Autodesk Inventor part; units mm, degrees
ref_plane "YZ Plane" through (0, 0, 0) normal (1, 0, 0) x (0, 1, 0)
ref_plane "XZ Plane" through (0, 0, 0) normal (0, 1, 0) x (-1, 0, 0)
ref_plane "XY Plane" through (0, 0, 0) normal (0, 0, 1) x (1, 0, 0)
sketch "Sketch1" plane through (0, 0, 0) normal (0, 1, 0) x (-1, 0, 0)
  line L0 (-3.5, -2.0207) -> (-3.5, 2.0207)
  line L1 (-3.5, 2.0207) -> (0, 4.0415)
  line L2 (0, 4.0415) -> (3.5, 2.0207)
  line L3 (3.5, 2.0207) -> (3.5, -2.0207)
  line L4 (3.5, -2.0207) -> (0, -4.0415)
  line L5 (0, -4.0415) -> (-3.5, -2.0207)
  point P0 (0, 0)
  point P1 (0, 0)
  dimension "d0" = 7
extrude "Extrusion1" add sketch "Sketch1" against normal blind 32
chamfer "Chamfer1" distance 0.1 angle 45 12 edges at (-1.75, -32, 3.0311) (1.75, -32, 3.0311) (3.5, -32, 0) (1.75, -32, -3.0311) (-1.75, -32, -3.0311) (-3.5, -32, 0) (1.75, 0, 3.0311) (-1.75, 0, 3.0311) (-3.5, 0, 0) (-1.75, 0, -3.0311) (1.75, 0, -3.0311) (3.5, 0, 0)
sketch "Sketch2" plane through (0, -32, 0) normal (0, -1, 0) x (1, 0, 0)
  circle A0 centre (0, 0) radius 2
  dimension "d6" = 4
extrude "Extrusion2" cut sketch "Sketch2" against normal blind 8
sketch "Sketch3" plane through (0, 0, 0) normal (0, 1, 0) x (1, 0, 0)
  circle A0 centre (0, 0) radius 2
  dimension "d9" = 4
extrude "Extrusion3" cut sketch "Sketch3" against normal blind 8
chamfer "Chamfer2" distance 0.2 angle 45 2 edges at (-2, 0, 0) (-2, -32, 0)
thread "Thread1"
thread "Thread2"
properties part number "09-0001" material "Aluminum 6061"
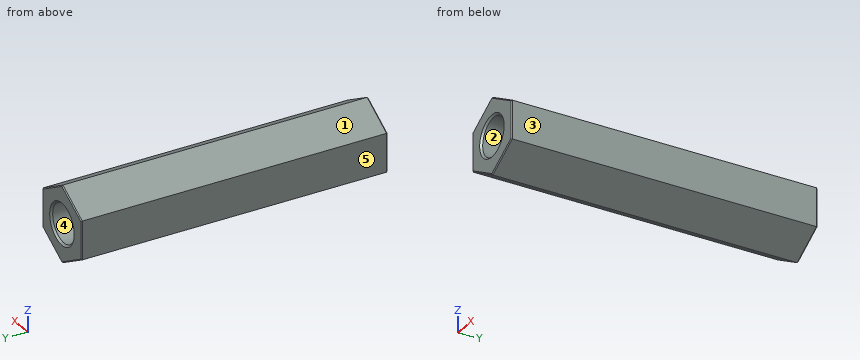
CAD build for the part. Positions are in the model's coordinates, mm. Face numbers are marked on the shaded views. A direction names the side the tool comes from. Round coordinates to 2 decimals unless told otherwise and drop trailing zeros. Order: outer loops, then holes, each group sorted by start corner. A loop starts at its lowest first (then second) coordinate and runs counter-clockwise, first axis right, second up. Notation, with made-up numbers: (13, 22) - (53, 22) arc R32 ccw to (53, 52) - close; hole circle Ø8 at (22.25, 7.5). An arc over 180 degrees is marked (long way). Return JSON: item names as keys, results as strings.
(1) Pin check, flat tips, straight feed: pin 1 Ø2 at (x, z) = (-0.5, -0.5) entering from +Y; pin 2 Ø3.5 at (x, z) = (0, 0) entering from -Y; pin 3 Ø1.5 at (x, y) = (-1.5, -16) entering from -Z. Stop position of each tip, or through.
Answer key:
{"pin 1": "stops at y = -8", "pin 2": "stops at y = -24", "pin 3": "stops at z = -3.61"}
(2) Pull direction X, two halves, no side cores. Call the marked faces 3, 4 and 5: +X half, -X half, draft (parallel to the pull), parting line (faces both ways), or undercut.
Answer key:
{"face 3": "+X half", "face 4": "undercut", "face 5": "-X half"}
(3) Cut at C-C (y = -8.5). Give the cut face in (x, z).
Answer key:
{"outline": "(-3.5, -2.02) - (0, -4.04) - (3.5, -2.02) - (3.5, 2.02) - (0, 4.04) - (-3.5, 2.02) - close"}
(4) Cut at B-B (z = 0). Give the cut face in (x, y), then the cut area to 3 significant figures.
Answer key:
{"outline": "(-3.5, -31.9) - (-3.4, -32) - (-2.2, -32) - (-2, -31.8) - (-2, -24) - (2, -24) - (2, -31.8) - (2.2, -32) - (3.4, -32) - (3.5, -31.9) - (3.5, -0.1) - (3.4, 0) - (2.2, 0) - (2, -0.2) - (2, -8) - (-2, -8) - (-2, -0.2) - (-2.2, 0) - (-3.4, 0) - (-3.5, -0.1) - close", "area": "160 mm^2"}
(5) Tool access for the marked faces 1 and 2: list every direction of +Z, -Z, +X, -X, +Y, -Y with a clear straight run to the whole face (end or side of a thin tool).
Answer key:
{"face 1": "+Z, -X, +Y, -Y", "face 2": "-Y"}
(6) Wall check: probe 1 along X at (y, z) = (-2.25, 0); probe 2 along Y at (x, z) = (-1.25, -1.25); probe 3 along X at (y, z) = (-31, -1). Give the ranges that are in metal, low to high. Write a range as from..to.
Answer key:
{"probe 1": "x = -3.5..-2, 2..3.5", "probe 2": "y = -24..-8", "probe 3": "x = -3.5..-1.73, 1.73..3.5"}
(7) Cut at A-A (y = -2). Give the cut face in (x, z), then the cut area to 3 significant figures.
Answer key:
{"outline": "(-3.5, -2.02) - (0, -4.04) - (3.5, -2.02) - (3.5, 2.02) - (0, 4.04) - (-3.5, 2.02) - close; hole circle Ø4 at (0, 0)", "area": "29.9 mm^2"}
